Can you work these out from the model? Positions are in its coordinate system, mm. A direction names the side the tool comes from. Coordinates: 2 decimals unless noted, no trailing zeros. Loops run counter-clockwise (first coordinate to the right, second up) from the corner with the lowest first, then second, coordinate; pieces in that order, holes last. Notation, with made-up numbers: (86.5, -26) -> (143.5, -26) arc R14 cw to (143.5, -22) -> close; hole circle Ø10 at (-3, 12). An arc over 180 degrees is marked (long way). Use one line per item in the form item = value. Start each with the question number.
(1) I'm going to push flat-ended pins straight in: pin 1 (0.6 mm diameter, centred on y = 9, z = 1.5, fed in from +X); pin 2 (3.5 mm diameter, centred on x = -2.5, y = -7.5, fed in from +Z); pin 3 (0.8 mm diameter, centred on x = 6.5, z = 1.5, fed in from -Y); pin 4 (10 mm diameter, centred on x = 29, y = -25, fed in from +Z). Where does each tip first touch, or does it pass through?
(2) Imagine slicing it at A-A (y = 27). List the corners of the cut face in (x, z) for me, plus the area to 4 significant figures.
(3) Imagine slicing it at C-C (z = 0.45). State how many separate pieces and enclosed holes the cut face has, plus the area to 3 significant figures.
(4) Thinking about a two-plate mould opening in X: for faces 4 (the flat face through (28.17, 14.37, 1.49)), 5 (the flat face through (27.235, 14.775, 1.493)), 6 (the flat face through (-23.518, -0.216, 1.493)), 7 (the flat face through (21.23, 11.77, 1.49)), which applies, released by +X, released by -X, zero draft, split by the parting line, or undercut?
(5) Imagine slicing it at D-D (x = -30.5). List the corners of the cut face in (y, z) for me, plus the area to 3 significant figures.
(6) Imagine slicing it at B-B (y = -23). List the corners of the cut face in (x, z) for me, plus the area to 3 significant figures.
(7) On a 3-axis mill with a long thin cutter (end or side, diameter ignored), from which of +Z, -Z, +X, -X, +Y, -Y can I reach the whole of each face in a straight line? I mean faces 1 (the flat face through (-5.175, -14.651, 1.493)), 2 (the cylindrical face through (10.613, 35.549, 0.493)), 3 (the flat face through (3.35, -1.79, 1.49)). Say none if no direction works.
(8) I need wall thicknesses on line 1 (Y direction, x = 45, z = 0.4); line 2 (X direction, y = -6.5, z = 0.65); line 3 (Y direction, x = -53.2, z = 0.75). Which ranges of each line are inside material? Lowest first, please. Write a range as [from, to].
```python
from build123d import *

# Parameters (mm, degrees)
SKETCH_R     = 0.75
SKETCH_R_2   = 15
SKETCH_R_3   = 3
SKETCH_W     = 1.5
SKETCH_H     = 71
SKETCH_W_2   = 6.5
SKETCH_H_2   = 6.5
PAD_DEPTH    = 1
PAD001_DEPTH = 2


with BuildPart() as part:
    # Sketch → Pad (new body)
    with BuildSketch(Plane.XY):
        with BuildLine():
            Line((-54.5, 50), (-54.5, -50))
            ThreePointArc((-54.5, -50), (-53.914214, -51.414214), (-52.5, -52))
            Line((-52.5, -52), (52.5, -52))
            ThreePointArc((52.5, -52), (53.914214, -51.414214), (54.5, -50))
            Line((54.5, -50), (54.5, 50))
            ThreePointArc((54.5, 50), (53.914214, 51.414214), (52.5, 52))
            Line((52.5, 52), (-52.5, 52))
            ThreePointArc((-52.5, 52), (-53.914214, 51.414214), (-54.5, 50))
        make_face()
        with Locations((-53.2, 50.7)):
            Circle(SKETCH_R, mode=Mode.SUBTRACT)
        with Locations((-53.2, -50.7)):
            Circle(SKETCH_R, mode=Mode.SUBTRACT)
        with Locations((53.2, -50.7)):
            Circle(SKETCH_R, mode=Mode.SUBTRACT)
        with Locations((53.2, 50.7)):
            Circle(SKETCH_R, mode=Mode.SUBTRACT)
        with Locations((22.5, -23)):
            Circle(SKETCH_R_2, mode=Mode.SUBTRACT)
        with Locations((12.824393, 33.521584)):
            Circle(SKETCH_R_3, mode=Mode.SUBTRACT)
        with Locations((21.542665, 33.324928)):
            Circle(SKETCH_R_3, mode=Mode.SUBTRACT)
        with Locations((-44.25, 3.5)):
            Rectangle(SKETCH_W, SKETCH_H, mode=Mode.SUBTRACT)
        with Locations((43.024296, 18.756004)):
            Rectangle(SKETCH_W_2, SKETCH_H_2, mode=Mode.SUBTRACT)
        with Locations((42.950272, 33.221375)):
            Rectangle(SKETCH_W_2, SKETCH_H_2, mode=Mode.SUBTRACT)
    extrude(amount=PAD_DEPTH)

    # Sketch002 → Pad001 (join)
    with BuildSketch(Plane.XY):
        Polygon((-34.773251, -3), (-34.749931, -2.337135), (-32.266365, -2), (-14.521888, 1.618207), (-11, 1.792153), (-11, 3), (-10.590711, 4.262184), (-9.755771, 6), (-8, 8.77106), (-6, 11), (-3, 13), (0.374559, 14.713974), (2.2, 15.1), (4.455713, 15.401265), (6.786591, 15.401265), (9, 15.22211), (11.437481, 14.54372), (13, 13.75457), (14.38553, 12.771906), (16, 11.618343), (18, 10), (24.546326, 13.584305), (30, 16), (30.289629, 15.70633), (26, 13), (22.625736, 11), (19.304169, 9), (19.304169, 8.492273), (20.679504, 6.520093), (20.705454, 6.260595), (20.290258, 6.312495), (18.85984, 8.1), (17.692602, 7), (16, 5), (14.708381, 3), (13.255195, 0.51859), (12.667271, -1.261222), (11.79619, -4.363118), (11.64747, -6), (13.75081, -5.552886), (15.429233, -5), (18.4249, -4), (20.443256, -4), (20, -4.55433), (19, -5.467902), (17.793219, -6.430947), (16, -7.474626), (11.618122, -9.301063), (4.782028, -11.249263), (1, -12.236397), (-1, -12.793026), (-1.547702, -12.462527), (-0.623532, -11.427116), (-0.6, -10.9), (-1, -10.745091), (-1.8, -10.925249), (-6.248158, -12.696156), (-2.838245, -15.840145), (-3.4, -16.256224), (-7, -13), (-9.221251, -10), (-10.394289, -7.518017), (-11, -5.353436), (-11.584344, -2.590018), (-11.665963, -1.389038), (-24.521864, -3.237807), (-24.550348, -2.782077), (-23.425266, -2.369072), (-22.214733, -1.656995), (-22, -1), (-27.459188, -2), (-33.301292, -3), align=None)
        Polygon((-10, -1.335219), (-8, -1.407553), (-6.690357, -2), (-4.764454, -2.731958), (-3.311275, -3.510448), (-2, -4.288938), (2, -8), (2, -8.466834), (2, -8.70038), (0.29573, -9.245323), (-0.664407, -9.686468), (-2, -10.28331), (-5.257498, -11.528893), (-6.633207, -12.253425), (-8, -10.248709), (-9, -8), (-9.782376, -6), (-10, -4.410032), align=None, mode=Mode.SUBTRACT)
        Polygon((-9.476856, 2), (-9.476856, 3), (-8.70385, 4.620335), (-7.235143, 7.237054), (-5, 9.697773), (-3.364116, 11), (-1, 12.533089), (1.568817, 13.51206), (3.648072, 14), (4.4, 14.148623), (7.4, 14.148623), (8.464255, 14.148623), (10, 13.747993), (11, 13.469228), (12.048037, 13.1), (13.953865, 12.172708), (15.3, 11.346745), (17, 10.170516), (17.033005, 9.447416), (15.575068, 8.67393), (13.726978, 7.225599), (13, 6.481995), (12.600948, 6), (12, 5), (11, 3), (10.22023, 0.508264), (9.364268, -2.641001), (9, -3.782789), (9, -4.716979), (8.549188, -6), (-2, 2.543029), align=None, mode=Mode.SUBTRACT)
    extrude(amount=PAD001_DEPTH)


solid = part.part
```
Worked out:
q1.pin_1 = 19.8
q1.pin_2 = 1
q1.pin_3 = -10.87
q1.pin_4 = through
q2.outline = (-54.5, 0) -> (-45, 0) -> (-45, 1) -> (-54.5, 1) -> close; (-43.5, 0) -> (54.5, 0) -> (54.5, 1) -> (-43.5, 1) -> close
q2.area = 107.5 mm2
q3.separate_pieces = 1
q3.enclosed_holes = 10
q3.area = 10,400 mm2
q4.face_4 = released by +X
q4.face_5 = undercut
q4.face_6 = released by -X
q4.face_7 = undercut
q5.outline = (-52, 0) -> (52, 0) -> (52, 1) -> (-1.64, 1) -> (-1.64, 2) -> (-2.52, 2) -> (-2.52, 1) -> (-52, 1) -> close
q5.area = 105 mm2
q6.outline = (-54.5, 0) -> (-45, 0) -> (-45, 1) -> (-54.5, 1) -> close; (-43.5, 0) -> (7.5, 0) -> (7.5, 1) -> (-43.5, 1) -> close; (37.5, 0) -> (54.5, 0) -> (54.5, 1) -> (37.5, 1) -> close
q6.area = 77.5 mm2
q7.face_1 = +Z, -X, -Y
q7.face_2 = +Z, -Z
q7.face_3 = +Z
q8.line_1 = [-52, 15.51], [22.01, 29.97], [36.47, 52]
q8.line_2 = [-54.5, -45], [-43.5, 54.5]
q8.line_3 = [-51.87, -51.45], [-49.95, 49.95], [51.45, 51.87]
